Geometry check sheet. Reference: the model listing, model coordinates, mm. A direction names the side the tool comes from. Give positions to 0.01 mm unless a question says otherwise; leave off trailing zeros. Loops run counter-clockwise (first coordinate to the right, second up) from the corner with the lowest first, then second, coordinate; pieces in that order, holes last. Notation, with made-up numbers: (78.5, 54.5) -> (97.5, 54.5) arc R19 cw to (97.5, 81.5) -> close; hole circle Ø6 at (-4.5, 20). An arc over 180 degrees is marked (long way). One line per item, written item: value. Start each with the question number.
(1) Scan lines: line 1 along X through (y, z) = (8.5, -9); line 2 along Y through (x, z) = (-0.25, 0); line 3 along Z through (x, y) = (0.5, 3.5). Record each from-to range of solid material in increasing order. Write a range as from..to.
(2) Sectioned sample at B-B, the plane z = -9.5. Record the cut outline in (x, y).
(3) Draft check along Z on faces 1 (the face through (5.5, 8, -11)), 2 (the face through (3, 8, -16)), 3 (the face through (0, 16, 5)), 4 (the face through (-4, 8, 14)). Enter one of: pulls with the +Z half, pulls with the -Z half, needs draft (parallel to the pull), parting line crosses it, or undercut.
(4) Sectioned sample at A-A, the plane z = 0. Record the cut outline in (x, y).
(5) Sectioned sample at C-C, the plane x = 2. Record the cut outline in (y, z).
(6) Tool access check on faces 5 (the face through (4, 7, 8)), 6 (the face through (7, 8, -13)), 7 (the face through (-6, 8, -13)), 8 (the face through (0, 14, 5)), 9 (the face through (-3, 8, -14)). Record the directions out of +Z, -Z, +X, -X, +Y, -Y that give a thin tool (end or side, any length) a straight path to the whole face; none if there is none.
(7) Sectioned sample at D-D, the plane y = 15. State how many separate pieces and enclosed holes the cut face has, then the cut area to 3 significant figures.
(8) Gauge pin test, flat ends, axial feed: pin 1 Ø6 at (x, y) = (5, 2.5) entering from -Z; pin 2 Ø3.5 at (x, y) = (-4, 6) entering from +Z; pin 3 Ø0.5 at (x, y) = (4.5, 16.5) entering from +Z. Record the tip position at first contact, or that the pin passes through.
from build123d import *

# Parameters (mm, degrees)
EXTRUDE_7_DEPTH          = 7
EXTRUDE_START            = 7
SKETCH_11_W              = 5
SKETCH_11_H              = 16
EXTRUDE_8_DEPTH          = 10
EXTRUDE_10_DEPTH         = 17
CUT_EXTRUDE_1_DEPTH      = 26.869866641
CUT_EXTRUDE_1_DEPTH_BACK = 26.869866641
SKETCH_15_R              = 2
CUT_EXTRUDE_2_DEPTH      = 26.869866641
CUT_EXTRUDE_2_DEPTH_BACK = 26.869866641


with BuildPart() as part:
    # 草图8 → 凸台-拉伸7 (new body)
    with BuildSketch(Plane(origin=(0, 0, 0), x_dir=(1, 0, 0), z_dir=(0, 1, 0))):
        with BuildLine():
            Line((4.5, -16), (2.5, -16))
            Line((2.5, -16), (2.5, -17.82554347))
            ThreePointArc((2.5, -17.82554347), (0, -18), (-2.5, -17.82554347))
            Line((-2.5, -17.82554347), (-2.5, -16))
            Line((-2.5, -16), (-4.49639369, -16))
            Line((-4.49639369, -16), (-4.49639369, -14))
            Line((-4.49639369, -14), (-2.5, -14))
            Line((-2.5, -14), (-2.5, -13))
            Line((-2.5, -13), (-2.5, 13))
            Line((-2.5, 13), (-2.5, 14))
            Line((-2.5, 14), (-4.49639369, 14))
            Line((-4.49639369, 14), (-4.49639369, 16))
            Line((-4.49639369, 16), (-2.5, 16))
            Line((-2.5, 16), (-2.5, 17.82554347))
            ThreePointArc((-2.5, 17.82554347), (0, 18), (2.5, 17.82554347))
            Line((2.5, 17.82554347), (2.5, 16))
            Line((2.5, 16), (4.5, 16))
            Line((4.5, 16), (4.5, 14))
            Line((4.5, 14), (2.5, 14))
            Line((2.5, 14), (2.5, 13))
            Line((2.5, 13), (2.5, -13))
            Line((2.5, -13), (2.5, -14))
            Line((2.5, -14), (4.5, -14))
            Line((4.5, -14), (4.5, -16))
        make_face()
    extrude(amount=EXTRUDE_7_DEPTH)

    # 草图11 → 凸台-拉伸8 (add)
    with BuildSketch(Plane(origin=(0, 0, 0), x_dir=(1, 0, 0), z_dir=(0, 1, 0)).offset(EXTRUDE_START)):
        Rectangle(SKETCH_11_W, SKETCH_11_H)
    extrude(amount=EXTRUDE_8_DEPTH)

    # 草图14 → 凸台-拉伸10 (add)
    with BuildSketch(Plane(origin=(0, 0, 0), x_dir=(1, 0, 0), z_dir=(0, 1, 0))):
        with BuildLine():
            ThreePointArc((-2.5, -17.82554347), (-1.253039812, -17.9563329), (0, -18))
            Line((0, -18), (0, 18))
            ThreePointArc((0, 18), (-1.253039812, 17.9563329), (-2.5, 17.82554347))
            Line((-2.5, 17.82554347), (-2.5, 16))
            Line((-2.5, 16), (-4.49639369, 16))
            Line((-4.49639369, 16), (-4.49639369, 14))
            Line((-4.49639369, 14), (-2.5, 14))
            Line((-2.5, 14), (-2.5, 8))
            Line((-2.5, 8), (-5.5, 8))
            Line((-5.5, 8), (-5.5, 13))
            Line((-5.5, 13), (-7.5, 13))
            Line((-7.5, 13), (-7.5, -13))
            Line((-7.5, -13), (-5.5, -13))
            Line((-5.5, -13), (-5.5, -8))
            Line((-5.5, -8), (-2.5, -8))
            Line((-2.5, -8), (-2.5, -14))
            Line((-2.5, -14), (-4.49639369, -14))
            Line((-4.49639369, -14), (-4.49639369, -16))
            Line((-4.49639369, -16), (-2.5, -16))
            Line((-2.5, -16), (-2.5, -17.82554347))
        make_face()
        with BuildLine():
            Line((4.5, -14), (2.5, -14))
            Line((2.5, -14), (2.5, -8))
            Line((2.5, -8), (5.5, -8))
            Line((5.5, -8), (5.5, -13))
            Line((5.5, -13), (7.5, -13))
            Line((7.5, -13), (7.5, 13))
            Line((7.5, 13), (5.5, 13))
            Line((5.5, 13), (5.5, 8))
            Line((5.5, 8), (2.5, 8))
            Line((2.5, 8), (2.5, 14))
            Line((2.5, 14), (4.5, 14))
            Line((4.5, 14), (4.5, 16))
            Line((4.5, 16), (2.5, 16))
            Line((2.5, 16), (2.5, 17.82554347))
            ThreePointArc((2.5, 17.82554347), (1.253039812, 17.9563329), (0, 18))
            Line((0, 18), (0, -18))
            ThreePointArc((0, -18), (1.253039812, -17.9563329), (2.5, -17.82554347))
            Line((2.5, -17.82554347), (2.5, -16))
            Line((2.5, -16), (4.5, -16))
            Line((4.5, -16), (4.5, -14))
        make_face()
    extrude(amount=EXTRUDE_10_DEPTH)

    # 草图15 → 切除-拉伸1 (cut, two sides: drawn at the far end of the back side and taken through both)
    with BuildSketch(Plane(origin=(0, 0, 0), x_dir=(0, 0, -1), z_dir=(1, 0, 0)).offset(-CUT_EXTRUDE_1_DEPTH_BACK)):
        with Locations((0, 3.5)):
            Circle(SKETCH_15_R)
    extrude(amount=CUT_EXTRUDE_1_DEPTH + CUT_EXTRUDE_1_DEPTH_BACK, mode=Mode.SUBTRACT)

    # 草图17 → 切除-拉伸2 (cut, two sides: drawn at the far end of the back side and taken through both)
    with BuildSketch(Plane(origin=(0, 0, 0), x_dir=(0, 0, -1), z_dir=(1, 0, 0)).offset(-CUT_EXTRUDE_2_DEPTH_BACK)):
        with BuildLine():
            Line((-10.5, 16), (-1.75, 16))
            ThreePointArc((-1.75, 16), (-0.75, 15), (-1.75, 14))
            Line((-1.75, 14), (-10.5, 14))
            ThreePointArc((-10.5, 14), (-11.5, 15), (-10.5, 16))
        make_face()
        with BuildLine():
            Line((1.75, 14), (10.5, 14))
            ThreePointArc((10.5, 14), (11.5, 15), (10.5, 16))
            Line((10.5, 16), (1.75, 16))
            ThreePointArc((1.75, 16), (0.75, 15), (1.75, 14))
        make_face()
    extrude(amount=CUT_EXTRUDE_2_DEPTH + CUT_EXTRUDE_2_DEPTH_BACK, mode=Mode.SUBTRACT)


solid = part.part
Calculated:
1. line 1: x = -7.5..-5.5, -2.5..2.5, 5.5..7.5
1. line 2: y = 0..1.5, 5.5..17
1. line 3: z = -17.99..-2, 2..17.99
2. outline: (-7.5, 0) -> (-5.5, 0) -> (-5.5, 14) -> (-7.5, 14) -> close; (-7.5, 16) -> (-5.5, 16) -> (-5.5, 17) -> (-7.5, 17) -> close; (-2.5, 0) -> (2.5, 0) -> (2.5, 14) -> (-2.5, 14) -> close; (-2.5, 16) -> (2.5, 16) -> (2.5, 17) -> (-2.5, 17) -> close; (5.5, 0) -> (7.5, 0) -> (7.5, 14) -> (5.5, 14) -> close; (5.5, 16) -> (7.5, 16) -> (7.5, 17) -> (5.5, 17) -> close
3. face 1: needs draft
3. face 2: pulls with the -Z half
3. face 3: undercut
3. face 4: undercut
4. outline: (-7.5, 0) -> (7.5, 0) -> (7.5, 1.5) -> (-7.5, 1.5) -> close; (-7.5, 5.5) -> (7.5, 5.5) -> (7.5, 17) -> (-7.5, 17) -> close
5. outline: (0, -17.89) -> (17, -17.89) -> (17, 17.89) -> (0, 17.89) -> close; hole circle Ø4 at (3.5, 0); hole (14, -10.5) arc R1 ccw to (16, -10.5) -> (16, -1.75) arc R1 ccw to (14, -1.75) -> close; hole (14, 1.75) arc R1 ccw to (16, 1.75) -> (16, 10.5) arc R1 ccw to (14, 10.5) -> close
6. face 5: +Y, -Y
6. face 6: -Z, +X, +Y, -Y
6. face 7: -Z, -X, +Y, -Y
6. face 8: +X, -X
6. face 9: -X, +Y, -Y
7. separate pieces: 7
7. enclosed holes: 0
7. area: 115 mm2
8. pin 1: stops at z = -17.89
8. pin 2: stops at z = 17.86
8. pin 3: stops at z = 16
